from build123d import *

# Parameters (mm, degrees)
CIRPATTERN1_COUNT  = 8
SKETCH4_R          = 28
CUT_EXTRUDE1_DEPTH = 0.8


with BuildPart() as part:
    # Sketch1 → Revolve1 (revolve)
    with BuildSketch(Plane.XY):
        Polygon((-15, 47.5), (-5, 47.5), (-5, 46), (-2, 46), (-2, 49), (0, 49), (0, 26), (-5, 26), (-5, 42.8), (-15, 42.8), align=None)
    revolve(axis=Axis((0, 0, 0), (-1, 0, 0)))

    # Sketch3 → M4 Clearance Hole1 (revolve, cut)
    with BuildSketch(Plane(origin=(0, 0, 38), x_dir=(0, 0, -1), z_dir=(0, 1, 0))):
        Polygon((0, 0), (0, 22.442065486), (2.4, 21), (2.4, 0.025), (2.425, 0), align=None)
    m4_clearance_hole1 = revolve(axis=Axis((6.35, 0, 38), (-1, 0, 0)), mode=Mode.SUBTRACT)

    # CirPattern1: M4 Clearance Hole1 ×8 about axis
    cirpattern1_axis = Axis((0, 0, 0), (1, 0, 0))
    for i in range(1, CIRPATTERN1_COUNT):
        add(m4_clearance_hole1.rotate(cirpattern1_axis, i * 360 / CIRPATTERN1_COUNT), mode=Mode.SUBTRACT)

    # Sketch4 → Cut-Extrude1 (cut)
    with BuildSketch(Plane.ZY.offset(5)):
        Circle(SKETCH4_R)
    extrude(amount=-CUT_EXTRUDE1_DEPTH, mode=Mode.SUBTRACT)


solid = part.part
CAD build for the part. Positions are in the model's coordinates, mm. A direction names the side the tool comes from. Round coordinates to 2 decimals unless told otherwise and drop trailing zeros. Write each loop counter-clockwise with the first axis right and the second up, starting at its lowest first coordinate (ties: lowest second). Pieces come first, ordered by that corner, then holes. Notation, with made-up numbers: M 76.25,40.25 L 105.25,40.25 A19 ccw 105.25,64.25 Z; hole C 53.25,24.5 d3. An arc over 180 degrees is marked long. Put each result on its own line as item: value. Start each with the question number.
1) Pull direction X, two halves, no side cores. Call faces 1 (the cylindrical face through (-2.478, -40.398, -0.106)), 2 (the flat face through (-15, 39, -18)), 3 (the cylindrical face through (-3.48, -5.99, -45.61)): pulls with the +X half, pulls with the -X half, needs draft (parallel to the pull), parting line crosses it, or undercut.
2) Drill centre lines: probe 1 along Z at (x, y) = (-2.45, 0); probe 2 along Z at (x, y) = (-1, 28.5); probe 3 along Z at (x, y) = (-8.75, 0). Where is each one in solid material? Low to high. Write a range as [from, to].
3) Pin check, flat tips, straight feed: pin 1 Ø5 at (x, z) = (-10, 21) entering from +Y; pin 2 Ø2 at (y, z) = (-35.5, 36.5) entering from +X; pin 3 Ø5 at (x, z) = (-8.5, -33) entering from +Y; pin 4 Ø6 at (y, z) = (26.87, -26.87) entering from -X. Stop position of each tip, or through.
4) Saw through at A-A, the plane z = 17.5. Write the cut outline in (x, y).
5) Saw through at B-B, the plane y = -15.5. Write the cut outline in (x, z).
6) 3-axis set-ups, long thin cutter, end or side, ignore diameter. For faces 4 (the flat face through (-5, -25, -39)), 5 (the cylindrical face through (-2.129, -20.633, 15.821)), 6 (the flat face through (-5, 1, -29)): which of +Z, -Z, +X, -X, +Y, -Y reach the whole face in a straight line?
7) Saw through at C-C, the plane x = -12.5. Write the cut outline in (y, z).
8) Saw through at D-D, the plane z = 0. Count the separate pieces of the cut face and the enclosed holes in it, and give its area (3 significant figures).
Resolved:
1. face 1: needs draft
1. face 2: pulls with the -X half
1. face 3: undercut
2. probe 1: [-46, -40.4], [-35.6, -26], [26, 35.6], [40.4, 46]
2. probe 2: [-39.86, -28.63], [-25.11, 25.11], [28.63, 39.86]
2. probe 3: [-47.5, -42.8], [42.8, 47.5]
3. pin 1: y = 43.75
3. pin 2: through
3. pin 3: y = 36.41
3. pin 4: x = -5
4. outline: M -15,-44.16 L -5,-44.16 L -5,-42.54 L -2,-42.54 L -2,-45.77 L 0,-45.77 L 0,-19.23 L -4.2,-19.23 L -4.2,-21.86 L -5,-21.86 L -5,-39.06 L -15,-39.06 Z; M -15,39.06 L -5,39.06 L -5,21.86 L -4.2,21.86 L -4.2,19.23 L 0,19.23 L 0,45.77 L -2,45.77 L -2,42.54 L -5,42.54 L -5,44.16 L -15,44.16 Z
5. outline: M -15,-44.9 L -5,-44.9 L -5,-43.31 L -2,-43.31 L -2,-46.48 L 0,-46.48 L 0,-20.87 L -4.2,-20.87 L -4.2,-23.32 L -5,-23.32 L -5,-39.89 L -15,-39.89 Z; M -15,39.89 L -5,39.89 L -5,23.32 L -4.2,23.32 L -4.2,20.87 L 0,20.87 L 0,46.48 L -2,46.48 L -2,43.31 L -5,43.31 L -5,44.9 L -15,44.9 Z
6. face 4: none
6. face 5: +X, -X
6. face 6: -X
7. outline: C 0,0 d95; hole C 0,0 d85.6
8. separate pieces: 4
8. enclosed holes: 0
8. area: 255 mm²
